For this review, use the dimensioned drawing (mm, ordinates from the lowest corner) and the shaded views. A direction names the side the tool comes from. Give positions to 0.01 mm unless a question says otherwise; leave off trailing zeros. Loops run counter-clockwise (first coordinate to the right, second up) from the corner with the lowest first, then second, coordinate; pieces in that order, holes last. Notation, with made-up numbers: M -13.75,10.5 L 43.25,10.5 A32 cw 43.25,36.5 Z; hole C -31.5,88 d2. An arc over 180 degrees is marked long. Return JSON: item names as keys, results as strings.
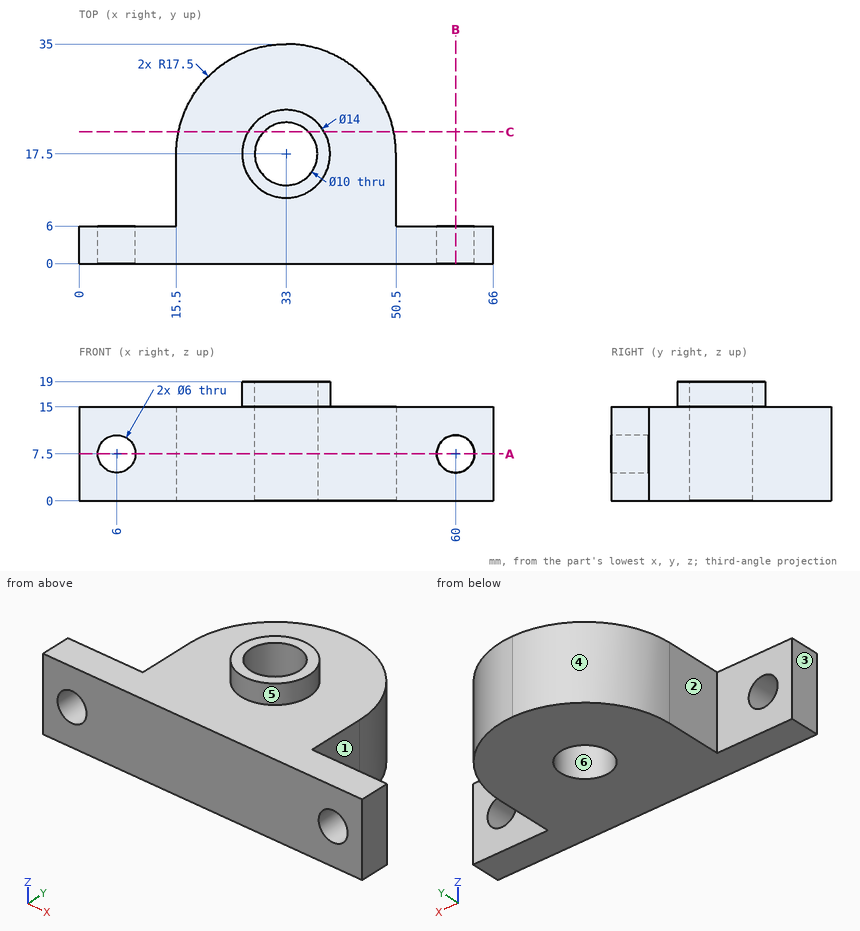
1) Consider section C-C on y = 21. Write out the cut boundary in (x, z).
From the geometry:
{"outline": "M 15.85,0 L 29.43,0 L 29.43,19 L 26.94,19 L 26.94,15 L 15.85,15 Z; M 36.57,0 L 50.15,0 L 50.15,15 L 39.06,15 L 39.06,19 L 36.57,19 Z"}
2) Wall thickness on L1, parallel to X at y = 3.05, z = 7.5; L2, parallel to Y at x = 33, z = 5; L3, parallel to Z at x = 60, y = 4.6: over which ranges is each line inside the solid? List them lowest first. Write a range as from..to.
From the geometry:
{"L1": "0..3, 9..57, 63..66", "L2": "0..12.5, 22.5..35", "L3": "0..4.5, 10.5..15"}
3) Consider section B-B on x = 60. Write out the cut boundary in (y, z), then the cut area to 3 significant figures.
From the geometry:
{"outline": "M 0,0 L 6,0 L 6,4.5 L 0,4.5 Z; M 0,10.5 L 6,10.5 L 6,15 L 0,15 Z", "area": "54.0 mm²"}
4) Insertion check: pin 1 (7.5 mm diameter, centred on x = 11, z = 4, fed in from +Y); pin 2 (3 mm diameter, centred on x = 25, y = 29.5, fed in from -Z); pin 3 (6 mm diameter, centred on y = 17, z = 13, fed in from -X); pin 4 (3.5 mm diameter, centred on y = 10.5, z = 7.5, fed in from +X). Each pin has a flat end and moves straight along its axis. Give the tip position at first contact, or say it passes through.
From the geometry:
{"pin 1": "y = 6", "pin 2": "z = 0", "pin 3": "x = 15.5", "pin 4": "x = 50.5"}
5) The part is to be moulded in two halves that separate along X. For the marked faces 4, 5 and 6, say which applies: released by +X, released by -X, zero draft, split by the parting line, or undercut.
From the geometry:
{"face 4": "released by -X", "face 5": "split by the parting line", "face 6": "undercut"}
6) Tool access review of the marked faces 1, 2 and 3: name each direction out of +Z, -Z, +X, -X, +Y, -Y from which nothing blocks a thin tool from reaching the whole face with its end or side.
From the geometry:
{"face 1": "+Z, -Z, +X, +Y", "face 2": "+Z, -Z, -X, +Y", "face 3": "+Z, -Z, -X, +Y, -Y"}
7) Consider section A-A on z = 7.5. Count the separate pieces of the cut face and the enclosed holes in it, then the cut area to 3 significant figures.
From the geometry:
{"separate pieces": "3", "enclosed holes": "1", "area": "1,130 mm²"}
